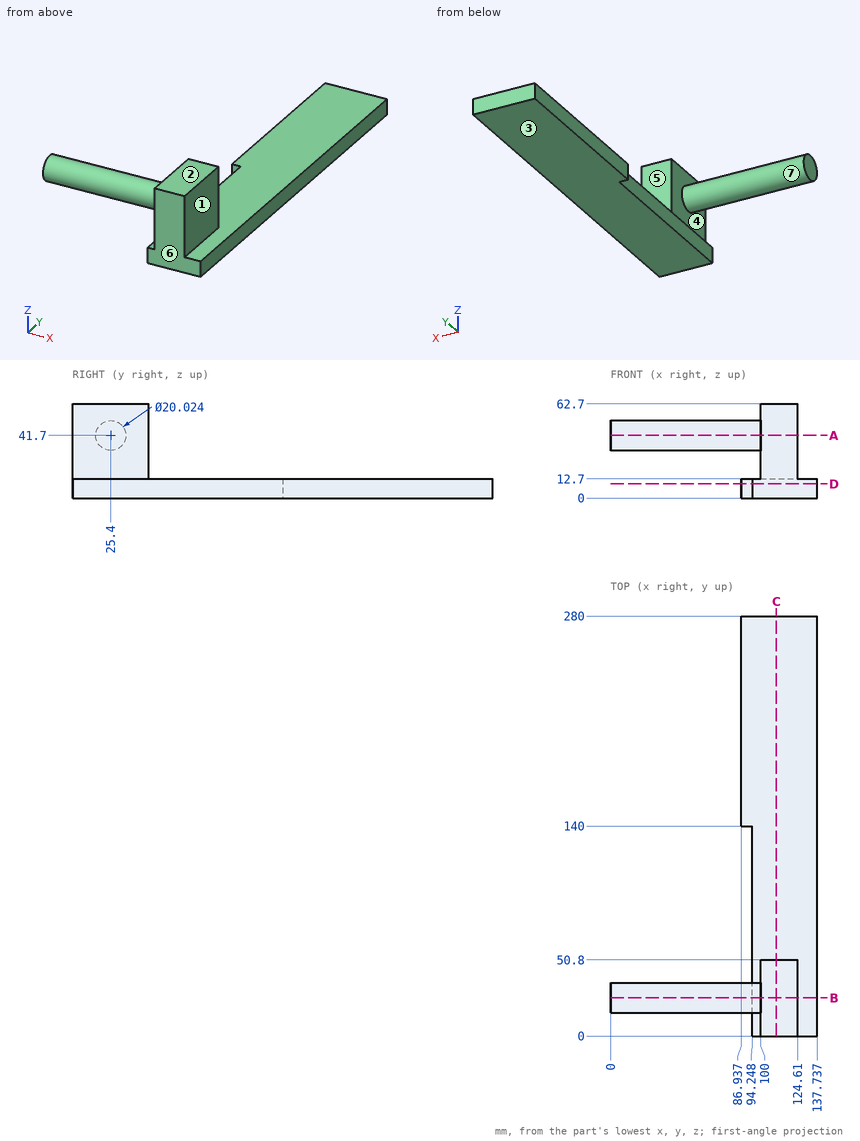
Geometry check sheet. Reference: drawing and pictorial views, mm from the part's lowest x, y, z. A direction names the side the tool comes from. Round coordinates to 2 decimals unless told otherwise and drop trailing zeros. Order: outer loops, then holes, each group sorted by start corner. A loop starts at its lowest first (then second) coordinate and runs counter-clockwise, first axis right, second up. Notation, with made-up numbers: M 19.25,-13 L 65.25,-13 A18 ccw 65.25,11 Z; hole C 79,88.5 d3. An arc over 180 degrees is marked long. Answer in a Markdown table with one row per item.
(1) Scan lines: probe 1 along Z at (x, y) = (109, 164); probe 2 along Y at (x, z) = (44, 42); probe 3 along X at (y, z) = (23.5, 18). Record each from-to range of solid material in increasing order. Write a range as from..to.
Responses:
| item | result |
|---|---|
| probe 1 | z = 0..12.7 |
| probe 2 | y = 15.39..35.41 |
| probe 3 | x = 100..124.61 |
(2) Sectioned sample at B-B, the plane y = 25.4. Record the cut outline in (x, z).
Responses:
| item | result |
|---|---|
| outline | M 0,31.69 L 100,31.69 L 100,12.7 L 94.25,12.7 L 94.25,0 L 137.74,0 L 137.74,12.7 L 124.61,12.7 L 124.61,62.7 L 100,62.7 L 100,51.71 L 0,51.71 Z |
(3) Go/stop test with flat-tipped pins: P1, Ø6, axis at x = 90, z = 5.5, coming from the -Y side; P2, Ø12, axis at y = 41.5, z = 33, coming from the +X side; P3, Ø14, axis at y = 175.5, z = 9, coming from the -X side. Record where each tip stops, or that it passes through.
Responses:
| item | result |
|---|---|
| P1 | stops at y = 140 |
| P2 | stops at x = 124.61 |
| P3 | stops at x = 86.94 |
(4) Draft check along Z on the marked faces 1, 2, 3 and 4. Enter one of: released by +Z, released by -Z, zero draft, split by the parting line, or undercut.
Responses:
| item | result |
|---|---|
| face 1 | zero draft |
| face 2 | released by +Z |
| face 3 | released by -Z |
| face 4 | undercut |
(5) Sectioned sample at A-A, the plane z = 41.7. Record the cut outline in (x, y).
Responses:
| item | result |
|---|---|
| outline | M 0,15.39 L 100,15.39 L 100,0 L 124.61,0 L 124.61,50.8 L 100,50.8 L 100,35.41 L 0,35.41 Z |
(6) Sectioned sample at D-D, the plane z = 9.5. Record the cut outline in (x, y), and give its area (3 significant figures).
Responses:
| item | result |
|---|---|
| outline | M 86.94,140 L 94.25,140 L 94.25,0 L 137.74,0 L 137.74,280 L 86.94,280 Z |
| area | 13,200 mm² |
(7) Tool access check on the marked faces 5, 6 and 7. Record the directions out of +Z, -Z, +X, -X, +Y, -Y that give a thin tool (end or side, any length) a straight path to the whole face; none if there is none.
Responses:
| item | result |
|---|---|
| face 5 | +Z, +X, -X, +Y |
| face 6 | +Z, -Z, +X, -X, -Y |
| face 7 | -X |
(8) Sectioned sample at C-C, the plane x = 110.5. Record the cut outline in (y, z), and give its area (3 significant figures).
Responses:
| item | result |
|---|---|
| outline | M 0,0 L 280,0 L 280,12.7 L 50.8,12.7 L 50.8,62.7 L 0,62.7 Z |
| area | 6,100 mm² |
